Autodesk Inventor part; units mm, degrees
ref_plane "YZ Plane" through (0, 0, 0) normal (1, 0, 0) x (0, 1, 0)
ref_plane "XZ Plane" through (0, 0, 0) normal (0, 1, 0) x (-1, 0, 0)
ref_plane "XY Plane" through (0, 0, 0) normal (0, 0, 1) x (1, 0, 0)
sketch "Sketch1" plane through (0, 0, 0) normal (1, 0, 0) x (0, 1, 0)
  circle A0 centre (0, 0) radius 12.7
  dimension "d0" = 25.4
extrude "Extrusion1" add sketch "Sketch1" along normal blind 19.05
sketch "Sketch2" plane through (19.05, 0, 0) normal (1, 0, 0) x (0, 0, -1)
  circle A0 centre (0, 0) radius 11.1125
  dimension "d3" = 22.225
extrude "Extrusion2" cut sketch "Sketch2" against normal blind 15.875
sketch "Sketch3" plane through (3.175, 0, 0) normal (1, 0, 0) x (0, 0, -1)
  circle A0 centre (0, 0) radius 3.175
  dimension "d6" = 6.35
extrude "Extrusion3" add sketch "Sketch3" along normal blind 22.225
sketch "Sketch4" plane through (0, 0, 0) normal (0, 1, 0) x (-1, 0, 0)
  circle A0 centre (-22.225, 0) radius 1.5875
  line L0 (-25.4, 3.175) -> (-25.4, -3.175)
  point P0 (0, 0)
  dimension "d9" = 3.175
  dimension "d10" = 3.175
extrude "Extrusion4" cut sketch "Sketch4" against normal mid plane 22.225
chamfer "Chamfer1" distance 0.7937 angle 45 2 edges at (19.05, -12.7, 0) (25.4, 0, 3.175)
Geometry: final body of the model. Coordinates: model frame, mm. A direction names the side the tool comes from. Give positions to 0.01 mm unless a question says otherwise; leave off trailing zeros. Write each loop counter-clockwise with the first axis right and the second up, starting at its lowest first coordinate (ties: lowest second). Pieces come first, ordered by that corner, then holes. Notation, with made-up numbers: M 41,32.5 L 47,32.5 A12 ccw 47,36.5 Z; hole C 30.5,54.5 d3. An arc over 180 degrees is marked long. Answer in a Markdown table with one row per item. Add a question column.
(1) Mould query, pull axis Z, two halves, no side actions, for faces 3 (the flat face through (0, 0, 0)), 4 (the cylindrical face through (21.372, 0.044, 1.339)), 5 (the cylindrical face through (9, -2.75, 12.4)). Classes: +Z half, -Z half, draft (parallel to the pull), parting line (faces both ways), or undercut.
(2) Section C-C on x = 9. State how many separate pieces and enclosed holes the cut face has, and give its area (3 significant figures).
(3) Reachability of faces 1 (the flat face through (25.4, 0, 0)), 2 (the cylindrical face through (13.74, -0.95, -3.03)) from +Z, -Z, +X, -X, +Y, -Y: full face, straight path, thin tool, end or side. Return the list, or none.
(4) Section D-D on x = 21.75. Return loops of the section in (y, z) (3 decimals), and give its area (3 significant figures).
(5) Ray query, line 1 (Z direction, x = 4.25, y = -1); line 2 (Z direction, x = 8.5, y = -1.25). Return the intervals inside material, ascending.
(6) First-contact query: pin 1 (1.5 mm diameter, centred on x = 7.5, z = 4, fed in from +Y); pin 2 (1.5 mm diameter, centred on x = 9, y = 7.5, fed in from -Z); pin 3 (1.5 mm diameter, centred on x = 5.5, y = -6, fed in from +Z). Flat tips, straight axial feed; report the tip coordinate or a pass-through.
Result set:
| question | item | result |
|---|---|---|
| 1 | face 3 | draft |
| 1 | face 4 | undercut |
| 1 | face 5 | parting line |
| 2 | separate pieces | 2 |
| 2 | enclosed holes | 1 |
| 2 | area | 150 mm^2 |
| 3 | face 1 | +Z, -Z, +X, +Y, -Y |
| 3 | face 2 | +X |
| 4 | outline | M -2.79,-1.515 A3.175 ccw 2.79,-1.515 Z; M -2.79,1.515 L 2.79,1.515 A3.175 ccw Z |
| 4 | area | 13.2 mm^2 |
| 5 | line 1 | z = -12.66 to -11.07, -3.01 to 3.01, 11.07 to 12.66 |
| 5 | line 2 | z = -12.64 to -11.04, -2.92 to 2.92, 11.04 to 12.64 |
| 6 | pin 1 | stops at y = 12.28 |
| 6 | pin 2 | stops at z = -10.76 |
| 6 | pin 3 | stops at z = 11.56 |
